Here's how the part is built. I have some questions about the finished solid (model axes, mm). Face numbers are marked on the shaded views. A direction names the side the tool comes from. Give positions to 0.01 mm unless a question says otherwise; leave off trailing zeros. Loops run counter-clockwise (first coordinate to the right, second up) from the corner with the lowest first, then second, coordinate; pieces in that order, holes last. Notation, with made-up numbers: (-40, -33.5) - (15, -33.5) arc R21 cw to (15, 3.5) - close; hole circle Ø7 at (-5.5, 68.5). An arc over 180 degrees is marked (long way). Use a Markdown table: item, result.
from build123d import *

# Parameters (mm, degrees)
SKETCH1_R                       = 3
SKETCH1_R_2                     = 1
BOSS_EXTRUDE1_DEPTH             = 9
SKETCH2_R                       = 8
CUT_EXTRUDE1_DEPTH              = 4
CIRPATTERN1_OUTLINE_R           = 1
CIRPATTERN1_DEPTH               = 5
TAP_DRILL_FOR_M3X0_5_TAP1_D     = 2.5
TAP_DRILL_FOR_M3X0_5_TAP1_DEPTH = 4
TAP_DRILL_FOR_M3X0_5_TAP1_TIP   = 0.751075774
SKETCH5_R                       = 1
CUT_EXTRUDE2_DEPTH              = 4
CHAMFER1_SIZE                   = 1


# Read off the part's stored shape, not the designer's step: CirPattern1
with BuildPart() as part:
    # Sketch1 → Boss-Extrude1 (new body)
    with BuildSketch(Plane(origin=(0, 0, 0), x_dir=(0, 0, -1), z_dir=(1, 0, 0))):
        with BuildLine():
            Line((0, 13), (0, 0))
            Line((0, 0), (14, 0))
            Line((14, 0), (14, 13))
            ThreePointArc((14, 13), (7, 20), (0, 13))
        make_face()
        with Locations((7, 13)):
            Circle(SKETCH1_R, mode=Mode.SUBTRACT)
        with Locations((12, 13)):
            Circle(SKETCH1_R_2, mode=Mode.SUBTRACT)
    extrude(amount=BOSS_EXTRUDE1_DEPTH)

    # Sketch2 → Cut-Extrude1 (cut)
    with BuildSketch(Plane(origin=(9, 0, 0), x_dir=(0, 0, -1), z_dir=(1, 0, 0))):
        with Locations((7, 13)):
            Circle(SKETCH2_R)
    extrude(amount=-CUT_EXTRUDE1_DEPTH, mode=Mode.SUBTRACT)

    # CirPattern1 outline → CirPattern1 (cut)
    with BuildSketch(Plane.YZ):
        with Locations((8, -7)):
            Circle(CIRPATTERN1_OUTLINE_R)
        with Locations((13, -2)):
            Circle(CIRPATTERN1_OUTLINE_R)
        with Locations((18, -7)):
            Circle(CIRPATTERN1_OUTLINE_R)
    extrude(amount=CIRPATTERN1_DEPTH, mode=Mode.SUBTRACT)

    # Tap Drill for M3x0.5 Tap1
    with Locations(Plane(origin=(0, 0, 0), x_dir=(-1, 0, 0), z_dir=(0, -1, 0))):
        with Locations((-3, 11), (-7, 3)):
            Hole(TAP_DRILL_FOR_M3X0_5_TAP1_D / 2, depth=TAP_DRILL_FOR_M3X0_5_TAP1_DEPTH)
            with Locations((0, 0, -(TAP_DRILL_FOR_M3X0_5_TAP1_DEPTH + TAP_DRILL_FOR_M3X0_5_TAP1_TIP / 2))):  # 118° drill point
                Cone(0, TAP_DRILL_FOR_M3X0_5_TAP1_D / 2, TAP_DRILL_FOR_M3X0_5_TAP1_TIP, mode=Mode.SUBTRACT)

    # Sketch5 → Cut-Extrude2 (cut)
    with BuildSketch(Plane.XZ):
        with Locations(Location((3, -3, 0), (0, 0, 270))):
            Circle(SKETCH5_R)
        with Locations(Location((7, -11, 0), (0, 0, 270))):
            Circle(SKETCH5_R)
    extrude(amount=-CUT_EXTRUDE2_DEPTH, mode=Mode.SUBTRACT)

    # Chamfer1
    chamfer1_edges = [part.edges().sort_by_distance(p)[0] for p in [
        (0, 13, -11),
        (0, 17, -7),
        (0, 12, -2),
        (0, 7, -7),
    ]]
    chamfer(chamfer1_edges, length=CHAMFER1_SIZE - 0.0001)  # a hair under: the kernel refuses the full size


solid = part.part
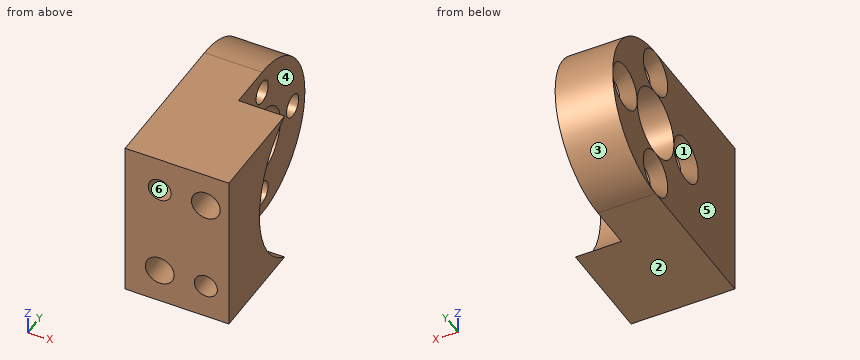
(1) Suppose I cut it at B-B on y = 5.5. Write out the boundary of the cut face in (x, z).
A:
| item | result |
|---|---|
| outline | (0, -14) - (9, -14) - (9, -9.78) - (5, -9.78) - (5, -4.22) - (9, -4.22) - (9, 0) - (0, 0) - close |
(2) On a 3-axis mill with a long thin cutter (end or side, diameter ignored), from which of +Z, -Z, +X, -X, +Y, -Y can I reach the whole of each face in a straight line? I mean the marked faces 4, 5 and 6. Say none if no direction works.
A:
| item | result |
|---|---|
| face 4 | +X, +Y |
| face 5 | +Z, -Z, -X, +Y, -Y |
| face 6 | -Y |
(3) We'd pull the mould along Z, two halves only. Please class the marked faces 1, 2 and 3: pulls with the +Z half, pulls with the -Z half, needs draft (parallel to the pull), parting line crosses it, or undercut.
A:
| item | result |
|---|---|
| face 1 | undercut |
| face 2 | pulls with the -Z half |
| face 3 | parting line crosses it |
(4) Suppose I cut it at A-A on y = 18. Write out the boundary of the cut face in (x, z), plus the area to 3 significant figures.
A:
| item | result |
|---|---|
| outline | (0, -11.9) - (5, -11.9) - (5, -8) - (1, -8) - (0, -9) - close; (0, -5) - (1, -6) - (5, -6) - (5, -2.1) - (0, -2.1) - close |
| area | 38.0 mm2 |
(5) Will these pins go through, and if not, where does the flat tip stop? pin 1 (5 mm diameter, centred on y = 15, z = -4.5, fed in from +X); pin 2 (2.5 mm diameter, centred on y = 13, z = -2, fed in from -X); pin 3 (1.2 mm diameter, centred on x = 7, z = -11, fed in from +Y).
A:
| item | result |
|---|---|
| pin 1 | x = 5 |
| pin 2 | x = 0.75 |
| pin 3 | y = 6.45 |
(6) If I drill on line 1 (Z direction, x = 3.7, y = 13); line 2 (X direction, y = 1.3, z = -11); line 3 (Y direction, x = 2, z = -7.25), over which ranges is the centre line in solid material (lowest first)?
A:
| item | result |
|---|---|
| line 1 | -14 to -13, -11 to -10, -4 to -3, -1 to 0 |
| line 2 | 0 to 1.75, 4.25 to 6, 8 to 9 |
| line 3 | 0 to 7.03, 8.97 to 10.01, 15.99 to 17.03, 18.97 to 20 |
(7) Suppose I cut it at D-D on y = 8. Write out the boundary of the cut face in (x, z) (3 decimals).
A:
| item | result |
|---|---|
| outline | (0, -14) - (9, -14) - (9, -13.245) - (5, -13.245) - (5, -8) - (1, -8) - (0, -9) - close; (0, -5) - (1, -6) - (5, -6) - (5, -0.755) - (9, -0.755) - (9, 0) - (0, 0) - close |
(8) Suppose I cut it at C-C on z = -7.5. Count the separate pieces of the cut face and the enclosed holes in it, plus the area to 3 significant figures.
A:
| item | result |
|---|---|
| separate pieces | 4 |
| enclosed holes | 0 |
| area | 70.9 mm2 |
